Geometry: final body of the model. Coordinates: model frame, mm. A direction names the side the tool comes from. Give positions to 0.01 mm unless a question says otherwise; leave off trailing zeros. Write each loop counter-clockwise with the first axis right and the second up, starting at its lowest first coordinate (ties: lowest second). Pieces come first, ordered by that corner, then holes.
Autodesk Inventor part; units mm, degrees
ref_plane "YZ Plane" through (0, 0, 0) normal (1, 0, 0) x (0, 1, 0)
ref_plane "XZ Plane" through (0, 0, 0) normal (0, 1, 0) x (-1, 0, 0)
ref_plane "XY Plane" through (0, 0, 0) normal (0, 0, 1) x (1, 0, 0)
sketch "Sketch1" plane through (0, 0, 0) normal (0, 0, 1) x (1, 0, 0)
  line L0 (0, 12) -> (11.3374, 12)
  line L1 (11.3374, 12) -> (11.3374, -10)
  line L2 (11.3374, -10) -> (0, -10)
  line L3 (0, -10) -> (0, 12)
  line L4 (3.0233, 0) -> (3.0233, 6.25) construction
  circle A0 centre (3.0233, 6.25) radius 1.65
  line L5 (3.0233, 0) -> (0, 0) construction
  circle A1 centre (3.0233, -6.25) radius 1.65
  circle A2 centre (-6.0697, 0) radius 7.5
  point P0 (0, 4.4056)
  point P1 (0, -4.4056)
  dimension "d0" = 3.3
  dimension "d1" = 6.25
  dimension "d2" = 11.3375
  dimension "d3" = 9.093
  dimension "d4" = 15
  dimension "d8" = 12
  dimension "d9" = 10
extrude "Extrusion1" add sketch "Sketch1" along normal blind 3 contours L0 L1 L2 L3 A2
sketch "Sketch2" plane through (0, 0, 0) normal (0, 0, -1) x (-1, 0, 0)
  line L0 (-11.3374, 12) -> (0, 12)
  line L1 (0, 12) -> (-17.8374, 12)
  line L2 (-17.8374, 12) -> (-17.8374, 17)
  line L3 (-17.8374, 17) -> (0, 17)
  line L4 (0, 17) -> (0, 12)
  line L5 (-11.3374, -10) -> (-11.3374, 12)
  point P0 (0, 0)
  dimension "d10" = 6.5
  dimension "d11" = 5
extrude "Extrusion2" add sketch "Sketch2" against normal blind 3
sketch "Sketch3" plane through (0, 0, 0) normal (0, 0, -1) x (-1, 0, 0)
  line L0 (-17.8374, 17) -> (0, 17)
  line L1 (-17.8374, 17) -> (-10.8374, 17)
  line L2 (-10.8374, 17) -> (-10.8374, 14)
  line L3 (-10.8374, 14) -> (-17.8374, 14)
  line L4 (-17.8374, 14) -> (-17.8374, 17)
  point P0 (0, 0)
  dimension "d14" = 3
  dimension "d15" = 7
extrude "Extrusion3" add sketch "Sketch3" along normal blind 7
fillet "Fillet1" radius 3 3 edges at (11.3374, -10, 1.5) (0, -10, 1.5) (0, 17, 1.5)
fillet "Fillet2" radius 5 1 edges at (11.3374, 12, 1.5)
fillet "Fillet3" radius 2 1 edges at (17.8374, 12, 1.5)
fillet "Fillet4" radius 1 1 edges at (14.3374, 14, 0)
fillet "Fillet5" radius 0.5 2 edges at (17.8374, 15.5, -7) (10.8374, 15.5, -7)
properties part number "Beam breaker"
Q1. Section B-B on x = 1.75. Output: boundary loops of the cut face in (y, z), plus the area to 3 significant figures.
Filled sheet:
outline: (-9.73, 0) - (-7.3, 0) - (-7.3, 3) - (-9.73, 3) - close; (-5.2, 0) - (5.2, 0) - (5.2, 3) - (-5.2, 3) - close; (7.3, 0) - (16.73, 0) - (16.73, 3) - (7.3, 3) - close
area: 66.8 mm2
Q2. Pin query (flat end, axial travel): P1, Ø3, axis at x = 13, z = -3.5, coming from the -Y side; P2, Ø9, axis at x = 6.5, y = 7, coming from the -Z side; P3, Ø0.9, axis at y = -3, z = 1, coming from the +X side. Return the tip coordinate at first contact, or that it passes through.
Filled sheet:
P1: stops at y = 14
P2: stops at z = 0
P3: stops at x = 11.34
Q3. Section D-D on x = 13.25. Output: boundary loops of the cut face in (y, z), plus the area to 3 significant figures.
Filled sheet:
outline: (10.93, 0) - (13, 0) arc R1 cw to (14, -1) - (14, -7) - (17, -7) - (17, 3) - (10.93, 3) - close
area: 39.4 mm2
Q4. Pull-direction query (Y, two-part tool) for faces 1 (the flat face through (11.337, 0, 1)), 2 (the cylindrical face through (2.67, 7.86, 1.48)), 3 (the cylindrical face through (14.288, 13.699, -0.285)); classes: released by +Y, released by -Y, zero draft, split by the parting line, or undercut.
Filled sheet:
face 1: zero draft
face 2: undercut
face 3: released by -Y
Q5. Ray query, line 1 along Y through (x, z) = (14.25, -2.5); line 2 along Y through (x, z) = (1.75, 2.5); line 3 along Z through (x, y) = (1, 10). Return the intervals inside material, ascending.
Filled sheet:
line 1: y = 14 to 17
line 2: y = -9.73 to -7.3, -5.2 to 5.2, 7.3 to 16.73
line 3: z = 0 to 3
Q6. Section C-C on z = 2. Count the separate pieces of the cut face and the enclosed holes in it, plus the area to 3 significant figures.
Filled sheet:
separate pieces: 1
enclosed holes: 2
area: 312 mm2
Q7. Access query for faces 4 (the cylindrical face through (10.44, -9.14, 1.52)), 5 (the flat face through (10.837, 15, -3)), 6 (the flat face through (14, 14, -4)). Directions: +Z, -Z, +X, -X, +Y, -Y. A direction counts if a zero-diameter tool reaches every point of the face in a straight line with its end or side. Return the directions, or none.
Filled sheet:
face 4: +Z, -Z, +X, -Y
face 5: -Z, -X, +Y, -Y
face 6: -Z, +X, -X, -Y
Q8. Section A-A on y = -6.25. Output: boundary loops of the cut face in (x, z), plus the area to 3 significant figures.
Filled sheet:
outline: (0, 0) - (1.37, 0) - (1.37, 3) - (0, 3) - close; (4.67, 0) - (11.34, 0) - (11.34, 3) - (4.67, 3) - close
area: 24.1 mm2
